Geometry check sheet. Reference: the model listing, model coordinates, mm. A direction names the side the tool comes from. Round coordinates to 2 decimals unless told otherwise and drop trailing zeros. Order: outer loops, then holes, each group sorted by start corner. A loop starts at its lowest first (then second) coordinate and runs counter-clockwise, first axis right, second up.
(1) Draft check along X on faces 1 (the face through (2, -64, 0)), 2 (the face through (1, -53, 0)), 3 (the face through (0, -64.484, 0)). Enter one of: pulls with the +X half, pulls with the -X half, needs draft (parallel to the pull), parting line crosses it, or undercut.
(2) Set-up check for faces 4 (the face through (0, -55, -5)), 5 (the face through (-1, -53, 0)), 6 (the face through (-0.9, -59.94, 2.86)): record each of +Z, -Z, +X, -X, +Y, -Y from which the full face is reachable in a straight line by a thin tool's end or side.
(3) Gauge pin test, flat ends, axial feed: P1, Ø3, axis at x = 3.5, y = -54.5, coming from the +Z side; P2, Ø0.6, axis at y = -53, z = 1, coming from the +X side; P3, Ø2, axis at y = -62, z = 2, coming from the +X side. Record the tip position at first contact, or that the pin passes through.
(4) Thickness scan on L1, parallel to Y at x = 1.5, z = 4; L2, parallel to Y at x = -0.5, z = 1.25; L3, parallel to Z at x = 1.5, y = -62.5. Record the ranges inside material, lowest first.
(5) Cross-section at B-B on y = -55.75. Enter the section's corners in (x, z), and give its area (3 significant figures).
(6) Cross-section at A-A on y = -61.75. Enter the section's corners in (x, z).
from build123d import *

# Parameters (mm, degrees)
CUT_EXTRUDE1_DEPTH      = 65.870739766
CUT_EXTRUDE1_DEPTH_BACK = 65.870739766
SKETCH2_W               = 2
SKETCH2_H               = 2


with BuildPart() as part:
    # Sketch1 → Revolve2 (revolve)
    with BuildSketch(Plane.XY, mode=Mode.PRIVATE) as revolve2_sk:
        with BuildLine():
            Line((0, -64.484206406), (2, -64.484206406))
            Line((2, -64.484206406), (2, -63.484206406))
            Line((2, -63.484206406), (3, -63.484206406))
            Line((3, -63.484206406), (3, -56.484206406))
            Line((3, -56.484206406), (5, -56.484206406))
            Line((5, -56.484206406), (5, -54.484206406))
            ThreePointArc((5, -54.484206406), (2.888936029, -52.33597969), (0, -51.484206406))
            Line((0, -51.484206406), (0, -64.44100966))
            Line((0, -64.44100966), (0, -64.484206406))
        make_face()
    revolve(revolve2_sk.sketch.rotate(Axis((0, 49.98015998, 0), (0, -1, 0)), 90), axis=Axis((0, 49.98015998, 0), (0, -1, 0)))

    # Sketch2 → Cut-Extrude1 (cut, two sides: drawn at the far end of the back side and taken through both)
    with BuildSketch(Plane.XY.offset(-CUT_EXTRUDE1_DEPTH_BACK)):
        with Locations((0, -52.484206406)):
            Rectangle(SKETCH2_W, SKETCH2_H)
    extrude(amount=CUT_EXTRUDE1_DEPTH + CUT_EXTRUDE1_DEPTH_BACK, mode=Mode.SUBTRACT)


solid = part.part
Found:
1. face 1: parting line crosses it
1. face 2: undercut
1. face 3: needs draft
2. face 4: +Y, -Y
2. face 5: +Z, -Z, +Y
2. face 6: -Y
3. P1: stops at z = 4.58
3. P2: stops at x = 3.99
3. P3: stops at x = 2.83
4. L1: y = -56.48 to -53.48
4. L2: y = -64.48 to -53.48
4. L3: z = -2.6 to 2.6
5. outline: circle Ø10 at (0, 0)
5. area: 78.5 mm2
6. outline: circle Ø6 at (0, 0)
